The model under review builds one solid part; all positions refer to its coordinate system, in mm. A direction names the side the tool comes from. Coordinates: 2 decimals unless noted, no trailing zeros. Loops run counter-clockwise (first coordinate to the right, second up) from the corner with the lowest first, then second, coordinate; pieces in that order, holes last. Notation, with made-up numbers: M 30,10 L 43,10 A32 ccw 43,36 Z; hole C 23.25,80 d6. An arc over 180 degrees is marked long. Use CSV: the item, a comma, the result in double quotes. Start each with the question number.
from build123d import *

# Parameters (mm, degrees)
F0_W     = 15.24
F0_H     = 25.4
F1_DEPTH = 5.08
F2_W     = 5.08
F2_H     = 5.08
F2_H_2   = 10.16
F3_DEPTH = 5.08
F4_SIZE  = 1.27


with BuildPart() as f1:
    # F0 (on Top) → F1 (new body)
    with BuildSketch(Plane.XY):
        Rectangle(F0_W, F0_H)
    extrude(amount=F1_DEPTH)

    # F2 (on face) → F3 (cut)
    with BuildSketch(Plane.XY.offset(5.08)):
        with Locations((0, 5.08)):
            Rectangle(F2_W, F2_H)
        with Locations((0, -7.62)):
            Rectangle(F2_W, F2_H_2)
    extrude(amount=-F3_DEPTH, mode=Mode.SUBTRACT)

    # F4
    f4_edges = [f1.edges().sort_by_distance(p)[0] for p in [
        (0, 7.62, 5.08),
        (0, 7.62, 0),
        (-2.54, 5.08, 5.08),
        (0, 2.54, 5.08),
        (2.54, 5.08, 5.08),
        (0, -2.54, 5.08),
        (-2.54, -7.62, 5.08),
        (2.54, -7.62, 5.08),
        (-7.62, 0, 5.08),
        (7.62, 0, 5.08),
        (0, 12.7, 5.08),
        (-5.08, -12.7, 5.08),
        (5.08, -12.7, 5.08),
        (-2.54, -12.7, 2.54),
        (2.54, -12.7, 2.54),
        (7.62, -12.7, 2.54),
        (-7.62, -12.7, 2.54),
        (-5.08, -12.7, 0),
        (5.08, -12.7, 0),
        (-7.62, 0, 0),
        (7.62, 0, 0),
        (-2.54, -7.62, 0),
        (2.54, -7.62, 0),
        (0, -2.54, 0),
        (0, 12.7, 0),
        (-2.54, 5.08, 0),
        (0, 2.54, 0),
        (2.54, 5.08, 0),
        (-7.62, 12.7, 2.54),
        (7.62, 12.7, 2.54),
    ]]
    chamfer(f4_edges, length=F4_SIZE)


solid = f1.part
1. Insertion check: pin 1 Ø5 at (x, y) = (-3.5, -1.5) entering from -Z; pin 2 Ø2 at (x, z) = (1, 2) entering from -Y. Each pin has a flat end and moves straight along its axis. Give the tip position at first contact, or say it passes through.
2. Add section C-C (z = 4.45). Write out the cut boundary in (x, y), plus the area to 3 significant figures.
3. Add section D-D (x = 5.75). Write out the cut boundary in (y, z).
4. To check wall thickness, follow line 1 along X through (y, z) = (4.75, 2.05); line 2 along Y through (x, z) = (-1.25, 4.6); line 3 along Y through (x, z) = (2, 0.6). State the ranges of each line that lie inside material, in increasing order.
5. Add section A-A (x = 1.25). Write out the cut boundary in (y, z).
6. Add section B-B (y = -10.25). Write out the cut boundary in (x, z).
7. For faces 4 (the flat face through (3.426, -11.831, 0.785)), 5 (the flat face through (-0.05, -1.91, 4.44)), 6 (the flat face through (3.17, -12.06, 2.56)), 7 (the flat face through (0, 2.54, 3)), list the 3-axis set-ups (+Z, -Z, +X, -X, +Y, -Y) from which the entire face can be reached by the end or side of a thin tool; tool diameter is ignored.
8. Draft analysis for pull direction X (two halves, no side actions). For faces 1 (the flat face through (0, 12.7, 3)), 2 (the flat face through (-6.98, -0.16, 0.63)), 3 (the flat face through (-0.05, 8.25, 4.44)), state which applies: released by +X, released by -X, zero draft, split by the parting line, or undercut.
Solved:
1,pin 1,"stops at z = 0"
1,pin 2,"stops at y = -2.54"
2,outline,"M -6.98,-11.43 L -6.35,-12.06 L -3.81,-12.06 L -3.18,-11.43 L -3.18,-1.9 L 3.18,-1.9 L 3.18,-11.43 L 3.81,-12.06 L 6.35,-12.06 L 6.98,-11.43 L 6.98,11.43 L 6.35,12.06 L -6.35,12.06 L -6.98,11.43 Z; hole M -3.18,1.9 L 3.18,1.9 L 3.18,8.26 L -3.18,8.26 Z"
2,area,"230 mm^2"
3,outline,"M -12.7,1.27 L -11.43,0 L 11.43,0 L 12.7,1.27 L 12.7,3.81 L 11.43,5.08 L -11.43,5.08 L -12.7,3.81 Z"
4,line 1,"x = -7.62 to -2.54, 2.54 to 7.62"
4,line 2,"y = -1.75 to 1.75, 8.41 to 11.91"
4,line 3,"y = -1.87 to 1.87, 8.29 to 12.03"
5,outline,"M -2.54,1.27 L -1.27,0 L 1.27,0 L 2.54,1.27 L 2.54,3.81 L 1.27,5.08 L -1.27,5.08 L -2.54,3.81 Z; M 7.62,1.27 L 8.89,0 L 11.43,0 L 12.7,1.27 L 12.7,3.81 L 11.43,5.08 L 8.89,5.08 L 7.62,3.81 Z"
6,outline,"M -7.62,1.27 L -6.35,0 L -3.81,0 L -2.54,1.27 L -2.54,3.81 L -3.81,5.08 L -6.35,5.08 L -7.62,3.81 Z; M 2.54,1.27 L 3.81,0 L 6.35,0 L 7.62,1.27 L 7.62,3.81 L 6.35,5.08 L 3.81,5.08 L 2.54,3.81 Z"
7,face 4,"-Z, -Y"
7,face 5,"+Z, -Y"
7,face 6,"+Z, -Z, -Y"
7,face 7,"+Z, -Z"
8,face 1,"zero draft"
8,face 2,"released by -X"
8,face 3,"undercut"
